```python
from build123d import *

# Parameters (mm, degrees)
SKETCH1_W           = 27.94
SKETCH1_H           = 114.3
BOSS_EXTRUDE1_DEPTH = 3
SKETCH2_R           = 1.2192
CUT_EXTRUDE1_DEPTH  = 59.90911135
LPATTERN1_COUNT     = 6
LPATTERN1_PITCH     = 21


with BuildPart() as part:
    # Sketch1 → Boss-Extrude1 (new body)
    with BuildSketch(Plane.XY):
        Rectangle(SKETCH1_W, SKETCH1_H)
    extrude(amount=BOSS_EXTRUDE1_DEPTH)

    # Sketch2 → Cut-Extrude1 (cut, through all)
    with BuildSketch(Plane.XY.offset(3)):
        with Locations((-9.9949, -54.15)):
            Circle(SKETCH2_R)
        with Locations((9.9949, -54.15)):
            Circle(SKETCH2_R)
    cut_extrude1 = extrude(amount=-CUT_EXTRUDE1_DEPTH, mode=Mode.SUBTRACT)

    # LPattern1: Cut-Extrude1 ×6
    with Locations(*[(0, i * LPATTERN1_PITCH, 0) for i in range(1, LPATTERN1_COUNT)]):
        add(cut_extrude1, mode=Mode.SUBTRACT)


solid = part.part
```
Could you check a few things on this model? Use its own coordinates, in mm. Round coordinates to 2 decimals unless told otherwise and drop trailing zeros. Loops run counter-clockwise (first coordinate to the right, second up) from the corner with the lowest first, then second, coordinate; pieces in that order, holes last. Notation, with made-up numbers: (12.5, 79) - (61.5, 79) arc R29 ccw to (61.5, 110) - close; hole circle Ø4 at (9, -26). An arc over 180 degrees is marked (long way). Answer in a Markdown table with one row per item. Add a question column.
(1) If we mould it in two halves opening along X, with no side actions, what happens to faces 1 (the face through (0, 57.15, 1)), 2 (the face through (-13.97, -1, 1)), 3 (the face through (-10.894, -11.326, 1.521))? For each: pulls with the +X half, pulls with the -X half, needs draft (parallel to the pull), parting line crosses it, or undercut.
(2) If we section it at A-A (y = 29.85): Please give me the cut outline in (x, z), plus the area to 3 significant figures.
(3) If we section it at C-C (z = 1.7): State how many separate pieces and enclosed holes the cut face has, plus the area to 3 significant figures.
(4) I need wall thicknesses on line 1 along X through (y, z) = (51, 1.45); line 2 along X through (y, z) = (-13, 2.5). Which ranges of each line are inside material? Lowest first, please.
(5) If we section it at B-B (x = 10): Please give me the cut outline in (y, z), plus the area to 3 significant figures.
Model answer:
| question | item | result |
|---|---|---|
| 1 | face 1 | needs draft |
| 1 | face 2 | pulls with the -X half |
| 1 | face 3 | undercut |
| 2 | outline | (-13.97, 0) - (-11.21, 0) - (-11.21, 3) - (-13.97, 3) - close; (-8.78, 0) - (8.78, 0) - (8.78, 3) - (-8.78, 3) - close; (11.21, 0) - (13.97, 0) - (13.97, 3) - (11.21, 3) - close |
| 2 | area | 69.2 mm² |
| 3 | separate pieces | 1 |
| 3 | enclosed holes | 12 |
| 3 | area | 3,140 mm² |
| 4 | line 1 | x = -13.97 to -11.2, -8.78 to 8.78, 11.2 to 13.97 |
| 4 | line 2 | x = -13.97 to -10.87, -9.12 to 9.12, 10.87 to 13.97 |
| 5 | outline | (-57.15, 0) - (-55.37, 0) - (-55.37, 3) - (-57.15, 3) - close; (-52.93, 0) - (-34.37, 0) - (-34.37, 3) - (-52.93, 3) - close; (-31.93, 0) - (-13.37, 0) - (-13.37, 3) - (-31.93, 3) - close; (-10.93, 0) - (7.63, 0) - (7.63, 3) - (-10.93, 3) - close; (10.07, 0) - (28.63, 0) - (28.63, 3) - (10.07, 3) - close; (31.07, 0) - (49.63, 0) - (49.63, 3) - (31.07, 3) - close; (52.07, 0) - (57.15, 0) - (57.15, 3) - (52.07, 3) - close |
| 5 | area | 299 mm² |
